Part model, mm, in its own coordinate system. Face numbers are marked on the shaded views. Round coordinates to 2 decimals unless told otherwise and drop trailing zeros. Order: outer loops, then holes, each group sorted by start corner. A loop starts at its lowest first (then second) coordinate and runs counter-clockwise, first axis right, second up. Notation, with made-up numbers: (-28, 3) - (17, 3) arc R17 ccw to (17, 27) - close; hole circle Ø5 at (21, -2). An arc over 180 degrees is marked (long way). Answer as a JSON object with one key per item and string values.
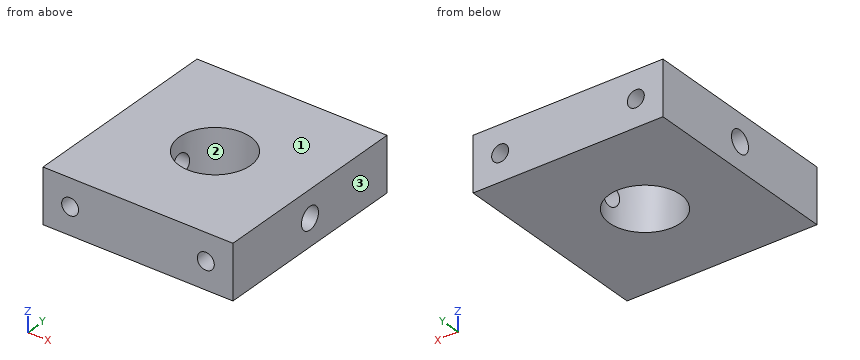
```python
from build123d import *

# Parameters (mm, degrees)
SKETCH_1_W             = 28
SKETCH_1_H             = 30
SKETCH_1_R             = 5.25
EXTRUDE_1_DEPTH        = 8
HOLE_WIZARD_M3_1_D     = 2.5
HOLE_WIZARD_M3_1_DEPTH = 11.5
HOLE_WIZARD_M3_1_TIP   = 0.751075774
HOLE_WIZARD_M3_2_D     = 2.5
HOLE_WIZARD_M3_2_DEPTH = 11.5
HOLE_WIZARD_M3_2_TIP   = 0.751075774
HOLE_WIZARD_M4_1_D     = 3.3


with BuildPart() as part:
    # 草图1 → 凸台-拉伸1 (new body)
    with BuildSketch(Plane.XY):
        Rectangle(SKETCH_1_W, SKETCH_1_H)
        Circle(SKETCH_1_R, mode=Mode.SUBTRACT)
    extrude(amount=EXTRUDE_1_DEPTH)

    # M3 螺纹孔1
    with Locations(Plane(origin=(0, 15, 0), x_dir=(1, 0, 0), z_dir=(0, 1, 0))):
        with Locations((-10, -4), (10, -4)):
            Hole(HOLE_WIZARD_M3_1_D / 2, depth=HOLE_WIZARD_M3_1_DEPTH)
            with Locations((0, 0, -(HOLE_WIZARD_M3_1_DEPTH + HOLE_WIZARD_M3_1_TIP / 2))):  # 118° drill point
                Cone(0, HOLE_WIZARD_M3_1_D / 2, HOLE_WIZARD_M3_1_TIP, mode=Mode.SUBTRACT)

    # M3 螺纹孔2
    with Locations(Plane(origin=(0, -15, 0), x_dir=(-1, 0, 0), z_dir=(0, -1, 0))):
        with Locations((10, -4), (-10, -4)):
            Hole(HOLE_WIZARD_M3_2_D / 2, depth=HOLE_WIZARD_M3_2_DEPTH)
            with Locations((0, 0, -(HOLE_WIZARD_M3_2_DEPTH + HOLE_WIZARD_M3_2_TIP / 2))):  # 118° drill point
                Cone(0, HOLE_WIZARD_M3_2_D / 2, HOLE_WIZARD_M3_2_TIP, mode=Mode.SUBTRACT)

    # M4 螺纹孔1 (through all)
    with Locations(Plane(origin=(14, 0, 0), x_dir=(0, 0, -1), z_dir=(1, 0, 0))):
        with Locations((-4, 0)):
            Hole(HOLE_WIZARD_M4_1_D / 2)


solid = part.part
```
Item 1: Probe L1, parallel to X at y = -12.5, z = 4; L2, parallel to X at y = 0, z = 5.75; L3, parallel to X at y = -5.75, z = 4.5. List the from-to ranges inside material, lowest first. Write a range as from..to.
Taken from the geometry:
{"L1": "-14..-11.25, -8.75..8.75, 11.25..14", "L2": "-14..-5.25, 5.25..14", "L3": "-14..-11.15, -8.85..8.85, 11.15..14"}
Item 2: Cut at B-B (x = 0). Write the cut outline in (y, z).
Taken from the geometry:
{"outline": "(-15, 0) - (-5.25, 0) - (-5.25, 8) - (-15, 8) - close; (5.25, 0) - (15, 0) - (15, 8) - (5.25, 8) - close"}
Item 3: Two-plate mould, pull along X, no slides. Class the marked faces 1, 2 and 3: pulls with the +X half, pulls with the -X half, needs draft (parallel to the pull), parting line crosses it, or undercut.
Taken from the geometry:
{"face 1": "needs draft", "face 2": "undercut", "face 3": "pulls with the +X half"}
Item 4: Cut at D-D (y = 4.75). Write the cut outline in (x, z).
Taken from the geometry:
{"outline": "(-14, 0) - (-2.24, 0) - (-2.24, 8) - (-14, 8) - close; (2.24, 0) - (14, 0) - (14, 8) - (2.24, 8) - close; hole circle Ø2.5 at (-10, 4); hole circle Ø2.5 at (10, 4)"}
Item 5: Cut at C-C (z = 1.5). Write the cut outline in (x, y).
Taken from the geometry:
{"outline": "(-14, -15) - (14, -15) - (14, 15) - (-14, 15) - close; hole circle Ø10.5 at (0, 0)"}
Item 6: Drop flat-ended pins along their axis: P1, Ø1.5, axis at x = -1.5, y = 4, coming from the -Z side; P2, Ø1.5, axis at x = -10, z = 4, coming from the -Y side; P3, Ø3, axis at x = 10, z = 4, coming from the +Y side; P4, Ø2, axis at x = -10, z = 4, coming from the +Y side. Give the stop position or say it passes through.
Taken from the geometry:
{"P1": "through", "P2": "y = -3.2", "P3": "y = 15", "P4": "y = 3.35"}
Item 7: Cut at A-A (y = 0). Write the cut outline in (x, z).
Taken from the geometry:
{"outline": "(-14, 0) - (-5.25, 0) - (-5.25, 2.35) - (-14, 2.35) - close; (-14, 5.65) - (-5.25, 5.65) - (-5.25, 8) - (-14, 8) - close; (5.25, 0) - (14, 0) - (14, 2.35) - (5.25, 2.35) - close; (5.25, 5.65) - (14, 5.65) - (14, 8) - (5.25, 8) - close"}
